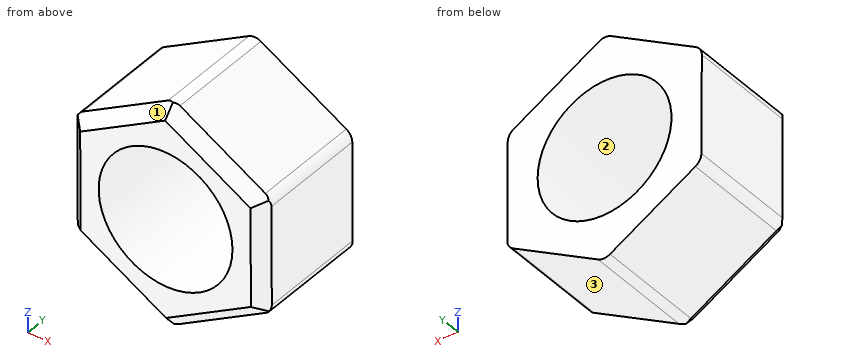
from build123d import *

# Parameters (mm, degrees)
F0_R     = 14.2875
F1_DEPTH = 25.4
F2_SIZE  = 2.54
F3_R     = 2.54


with BuildPart() as f1:
    # F0 (on Front) → F1 (new body)
    with BuildSketch(Plane.XZ):
        Polygon((20.667777, 12.055561), (-0.106534, 23.9266), (-20.774311, 11.871039), (-20.667777, -12.055561), (0.106534, -23.9266), (20.774311, -11.871039), align=None)
        Circle(F0_R, mode=Mode.SUBTRACT)
    extrude(amount=F1_DEPTH)

    # F2
    f2_edges = [f1.edges().sort_by_distance(p)[0] for p in [
        (-10.440422, -25.4, 17.89882),
        (-20.721044, -25.4, -0.092261),
        (-10.280621, -25.4, -17.991081),
        (10.440422, -25.4, -17.89882),
        (20.721044, -25.4, 0.092261),
        (10.280621, -25.4, 17.991081),
    ]]
    chamfer(f2_edges, length=F2_SIZE)

    # F3
    f3_edges = [f1.edges().sort_by_distance(p)[0] for p in [
        (-20.774311, -11.43, 11.871039),
        (-0.106534, -11.43, 23.9266),
        (-20.667777, -11.43, -12.055561),
        (0.106534, -11.43, -23.9266),
        (20.774311, -11.43, -11.871039),
        (20.667777, -11.43, 12.055561),
    ]]
    fillet(f3_edges, radius=F3_R)


solid = f1.part
Model file for the job. Use its own axes, mm. Face numbers are marked on the shaded views. Give positions to 0.01 mm unless a question says otherwise; leave off trailing zeros. Loops run counter-clockwise (first coordinate to the right, second up) from the corner with the lowest first, then second, coordinate; pieces in that order, holes last.
Item 1: Slice it at B-B (y = -20.5). Write the cut outline in (x, z) (1 decimal), plus the area to 3 significant figures.
Check values:
outline: (-20.8, 10.4) - (-20.7, -10.6) arc R2.5 ccw to (-19.4, -12.8) - (-1.2, -23.2) arc R2.5 ccw to (1.4, -23.2) - (19.5, -12.6) arc R2.5 ccw to (20.8, -10.4) - (20.7, 10.6) arc R2.5 ccw to (19.4, 12.8) - (1.2, 23.2) arc R2.5 ccw to (-1.4, 23.2) - (-19.5, 12.6) arc R2.5 ccw to start; hole circle Ø28.6 at (0, 0)
area: 844 mm2
Item 2: Drill centre lines: line 1 along Z through (x, y) = (0, -2); line 2 along Z through (x, y) = (10.5, -11.75); line 3 along X through (y, z) = (-11.5, 11.5). Where is each one in solid material? Low to high.
Check values:
line 1: z = -23.53 to -14.29, 14.29 to 23.53
line 2: z = -17.86 to -9.69, 9.69 to 17.87
line 3: x = -20.52 to -8.48, 8.48 to 20.5
Item 3: Slice it at A-A (z = 7). Write the cut outline in (x, y), plus the area to 3 significant figures.
Check values:
outline: (-20.75, -22.86) - (-18.21, -25.4) - (-12.46, -25.4) - (-12.46, 0) - (-20.75, 0) - close; (12.46, -25.4) - (18.15, -25.4) - (20.69, -22.86) - (20.69, 0) - (12.46, 0) - close
area: 413 mm2
Item 4: Mould opens along Z. For the marked faces 1, 2 and 3 say: +Z half, -Z half, draft (parallel to the pull), parting line (faces both ways), or undercut.
Check values:
face 1: +Z half
face 2: undercut
face 3: -Z half
Item 5: Slice it at C-C (x = -4). Write the cut outline in (y, z) (3 decimals).
Check values:
outline: (-25.4, -18.655) - (-22.86, -21.58) - (0, -21.58) - (0, -13.716) - (-25.4, -13.716) - close; (-25.4, 13.716) - (0, 13.716) - (0, 21.656) - (-22.86, 21.656) - (-25.4, 18.715) - close
Item 6: Drop flat-ended pins along their axis: P1, Ø6, axis at y = -9.5, z = 13, coming from the +X side; P2, Ø1.5, axis at y = -18.5, z = 4.5, coming from the -X side; P3, Ø1, axis at y = -4.5, z = -15.5, coming from the +X side. Give the stop position or say it passes through.
Check values:
P1: stops at x = 20.68
P2: stops at x = -20.74
P3: stops at x = 15.41
